Build history of the part. All positions in model axes, mm. A direction names the side the tool comes from. Coordinates: 2 decimals unless noted, no trailing zeros. Loops run counter-clockwise (first coordinate to the right, second up) from the corner with the lowest first, then second, coordinate; pieces in that order, holes last. Notation, with made-up numbers: (57, 39) - (114, 39) arc R12 cw to (114, 46) - close; hole circle Ø8 at (61.5, -2). An arc over 180 degrees is marked (long way). One line per item, written item: value.
```python
from build123d import *

# Parameters (mm, degrees)
SKETCH1_W         = 50
SKETCH1_H         = 45
BODY_DEPTH        = 0.5
CENTER_HOLE_DEPTH = 2
SKETCH3_R         = 3.5
HOLE_1_DEPTH      = 2
HOLES_2_4_COUNT   = 4
R4_FILLETS_R      = 4


with BuildPart() as part:
    # Sketch1 → Body (new body, symmetric)
    with BuildSketch(Plane(origin=(0, 0, 0), x_dir=(1, 0, 0), z_dir=(0, 1, 0))):
        with Locations((3, 0)):
            Rectangle(SKETCH1_W, SKETCH1_H)
    extrude(amount=BODY_DEPTH, both=True)

    # Sketch2 → Center hole (cut, through all)
    with BuildSketch(Plane(origin=(0, 0.5, 0), x_dir=(1, 0, 0), z_dir=(0, 1, 0))):
        with BuildLine():
            Line((17.88854382, 2), (24, 2))
            ThreePointArc((24, 2), (26, 0), (24, -2))
            Line((24, -2), (17.88854382, -2))
            ThreePointArc((17.88854382, -2), (-18, 0), (17.88854382, 2))
        make_face()
    extrude(amount=-CENTER_HOLE_DEPTH, mode=Mode.SUBTRACT)

    # Sketch3 → Hole 1 (cut, through all)
    with BuildSketch(Plane(origin=(0, 0.5, 0), x_dir=(1, 0, 0), z_dir=(0, 1, 0))):
        with Locations((16.263455967, 16.263455967)):
            Circle(SKETCH3_R)
    hole_1 = extrude(amount=-HOLE_1_DEPTH, mode=Mode.SUBTRACT)

    # Holes 2-4: Hole 1 ×4 about axis
    holes_2_4_axis = Axis((0, 0, 0), (0, 1, 0))
    for i in range(1, HOLES_2_4_COUNT):
        add(hole_1.rotate(holes_2_4_axis, i * 360 / HOLES_2_4_COUNT), mode=Mode.SUBTRACT)

    # R4 Fillets
    r4_fillets_edges = [part.edges().sort_by_distance(p)[0] for p in [
        (-22, 0, -22.5),
        (28, 0, -22.5),
        (28, 0, 22.5),
        (-22, 0, 22.5),
    ]]
    fillet(r4_fillets_edges, radius=R4_FILLETS_R)


solid = part.part
```
Item 1: Cut at C-C, the plane z = -17. Write the cut outline in (x, y), then the cut area to 3 significant figures.
Check result:
outline: (-22, -0.5) - (-19.69, -0.5) - (-19.69, 0.5) - (-22, 0.5) - close; (-12.84, -0.5) - (-5.92, -0.5) - (-5.92, 0.5) - (-12.84, 0.5) - close; (5.92, -0.5) - (12.84, -0.5) - (12.84, 0.5) - (5.92, 0.5) - close; (19.69, -0.5) - (28, -0.5) - (28, 0.5) - (19.69, 0.5) - close
area: 24.5 mm^2
Item 2: Tool access for faces 4 (the face through (26, 0, 0)), 5 (the face through (-20.859, 0.007, 21.297)): list every direction of +Z, -Z, +X, -X, +Y, -Y with a clear straight run to the whole face (end or side of a thin tool).
Check result:
face 4: +Y, -Y
face 5: +Z, -X, +Y, -Y
Item 3: Probe probe 1 along Z at (x, y) = (22, -0.2); probe 2 along Z at (x, y) = (0, -0.3); probe 3 along X at (y, z) = (-0.2, 0). List the from-to ranges inside material, lowest first. Write a range as from..to.
Check result:
probe 1: z = -22.5..-2, 2..22.5
probe 2: z = -22.5..-18, 18..22.5
probe 3: x = -22..-18, 26..28
Item 4: Cut at D-D, the plane y = 0.3. Write the cut outline in (x, z).
Check result:
outline: (-22, -18.5) arc R4 ccw to (-18, -22.5) - (24, -22.5) arc R4 ccw to (28, -18.5) - (28, 18.5) arc R4 ccw to (24, 22.5) - (-18, 22.5) arc R4 ccw to (-22, 18.5) - close; hole circle Ø7 at (-16.26, -16.26); hole circle Ø7 at (-16.26, 16.26); hole circle Ø7 at (16.26, -16.26); hole circle Ø7 at (16.26, 16.26); hole (17.89, -2) - (24, -2) arc R2 ccw to (24, 2) - (17.89, 2) arc R18 ccw (long way) to start
Item 5: Cut at A-A, the plane x = 0. Write the cut outline in (y, z).
Check result:
outline: (-0.5, -22.5) - (0.5, -22.5) - (0.5, -18) - (-0.5, -18) - close; (-0.5, 18) - (0.5, 18) - (0.5, 22.5) - (-0.5, 22.5) - close
Item 6: Pull direction X, two halves, no side cores. Call faces 1 (the face through (26.797, 0.007, 21.359)), 2 (the face through (19, -0.5, 5)), 3 (the face through (-13.16, 0.01, -17.88)): released by +X, released by -X, zero draft, split by the parting line, or undercut.
Check result:
face 1: released by +X
face 2: zero draft
face 3: undercut
Item 7: Cut at B-B, the plane z = 3. Write the cut outline in (x, y), then the cut area to 3 significant figures.
Check result:
outline: (-22, -0.5) - (-17.75, -0.5) - (-17.75, 0.5) - (-22, 0.5) - close; (17.75, -0.5) - (28, -0.5) - (28, 0.5) - (17.75, 0.5) - close
area: 14.5 mm^2
